Design review of the part built by this model. Coordinates are the model's own, in mm. A direction names the side the tool comes from. Round coordinates to 2 decimals unless told otherwise and drop trailing zeros. Write each loop counter-clockwise with the first axis right and the second up, starting at its lowest first coordinate (ties: lowest second). Pieces come first, ordered by that corner, then holes. Notation, with made-up numbers: M 21,16.25 L 70,16.25 A11 cw 70,21.25 Z; hole C 7.25,27.5 d5. An arc over 180 degrees is marked long. One line per question, with ' | ' between items. Start each with the question number.
Item 1: Machinability: for faces 1 (the face through (-11.986, 1.972, -1.586)), 2 (the face through (-2.645, 1.972, -13.127)), 3 (the face through (-11.15, 1.97, -7.41)), 4 (the face through (11.995, 1.972, -5.952)), which of the approach directions +Z, -Z, +X, -X, +Y, -Y give a long, thin tool a straight path to every point of the face, cutting with its end or side? Answer none if there is none.
Item 2: Insertion check: pin 1 Ø1 at (x, y) = (13.5, 1) entering from -Z; pin 2 Ø1.2 at (x, y) = (22.5, 1.5) entering from +Z; pin 3 Ø3.5 at (x, z) = (4.5, 0) entering from -Y; pin 4 Ø1 at (x, y) = (16, 1.5) entering from -Z. Each pin has a flat end and moves straight along its axis. Give the tip position at first contact, or say it passes through.
Item 3: Add section A-A, the plane y = 3.2. Give the number of separate pieces and of enclosed holes in the cut face, and give its area (3 significant figures).
Item 4: Add section B-B, the plane x = 19. State the section outline as (y, z) points.
Item 5: Draft analysis for pull direction X (two halves, no side actions). For faces 5 (the face through (10.046, 1.972, -8.853)), 6 (the face through (2.664, 1.972, -13.159)), 7 (the face through (-13.159, 1.972, -2.664)), state which applies: released by +X, released by -X, zero draft, split by the parting line, or undercut.
Item 6: For L1, parallel to X at y = 2.1, z = 0; L2, parallel to Z at x = 21, y = 3.3; L3, parallel to Z at x = -11.5, y = 1.75, list the stretches that pass through material, from the lowest coordinate up.
Item 7: Add section C-C, the plane z = -3. State the section outline as (x, y) points, and give its area (3 significant figures).
```python
from build123d import *

# Parameters (mm, degrees)
SKETCH_2_R          = 1.75
EXTRUDE_1_DEPTH     = 4
SKETCH_3_R          = 2.4
SKETCH_3_R_2        = 1.3
CUT_EXTRUDE_1_DEPTH = 38.993706757


with BuildPart() as part:
    # 草图2 → 凸台-拉伸1 (new body)
    with BuildSketch(Plane(origin=(0, 0, 0), x_dir=(1, 0, 0), z_dir=(0, 1, 0))):
        with BuildLine():
            ThreePointArc((30.75, -4.085109489), (34.835109489, 0), (30.75, 4.085109489))
            Line((30.75, 4.085109489), (14.048088143, 4.085109489))
            ThreePointArc((14.048088143, 4.085109489), (12.709169027, 4.272836063), (11.365584201, 4.122086336))
            ThreePointArc((11.365584201, 4.122086336), (11.169703548, 4.626642697), (10.951436862, 5.12192646))
            ThreePointArc((10.951436862, 5.12192646), (12.008090957, 5.965388247), (12.82210701, 7.044889767))
            ThreePointArc((12.82210701, 7.044889767), (12.669951657, 7.315), (12.51210701, 7.581825517))
            ThreePointArc((12.51210701, 7.581825517), (11.170223244, 7.416617696), (9.911436862, 6.9232593))
            ThreePointArc((9.911436862, 6.9232593), (9.591641884, 7.359925677), (9.252623584, 7.781841479))
            ThreePointArc((9.252623584, 7.781841479), (10.05496909, 8.870045207), (10.561852666, 10.123446462))
            ThreePointArc((10.561852666, 10.123446462), (10.344972209, 10.344972209), (10.123446462, 10.561852666))
            ThreePointArc((10.123446462, 10.561852666), (8.870045207, 10.05496909), (7.781841479, 9.252623584))
            ThreePointArc((7.781841479, 9.252623584), (7.359925677, 9.591641884), (6.9232593, 9.911436862))
            ThreePointArc((6.9232593, 9.911436862), (7.416617696, 11.170223244), (7.581825517, 12.51210701))
            ThreePointArc((7.581825517, 12.51210701), (7.315, 12.669951657), (7.044889767, 12.82210701))
            ThreePointArc((7.044889767, 12.82210701), (5.965388247, 12.008090957), (5.12192646, 10.951436862))
            ThreePointArc((5.12192646, 10.951436862), (4.626642697, 11.169703548), (4.122086336, 11.365584201))
            ThreePointArc((4.122086336, 11.365584201), (4.272836063, 12.709169027), (4.085109489, 14.048088143))
            ThreePointArc((4.085109489, 14.048088143), (3.78652263, 14.131494839), (3.486235477, 14.208555951))
            ThreePointArc((3.486235477, 14.208555951), (2.654199937, 13.14288127), (2.112960617, 11.903927815))
            ThreePointArc((2.112960617, 11.903927815), (1.578061664, 11.986568374), (1.04, 12.04518576))
            ThreePointArc((1.04, 12.04518576), (0.837867713, 13.382005944), (0.31, 14.626715284))
            ThreePointArc((0.31, 14.626715284), (0, 14.63), (-0.31, 14.626715284))
            ThreePointArc((-0.31, 14.626715284), (-0.837867713, 13.382005944), (-1.04, 12.04518576))
            ThreePointArc((-1.04, 12.04518576), (-1.578061664, 11.986568374), (-2.112960617, 11.903927815))
            ThreePointArc((-2.112960617, 11.903927815), (-2.654199937, 13.14288127), (-3.486235477, 14.208555951))
            ThreePointArc((-3.486235477, 14.208555951), (-3.78652263, 14.131494839), (-4.085109489, 14.048088143))
            ThreePointArc((-4.085109489, 14.048088143), (-4.272836063, 12.709169027), (-4.122086336, 11.365584201))
            ThreePointArc((-4.122086336, 11.365584201), (-4.626642697, 11.169703548), (-5.12192646, 10.951436862))
            ThreePointArc((-5.12192646, 10.951436862), (-5.965388247, 12.008090957), (-7.044889767, 12.82210701))
            ThreePointArc((-7.044889767, 12.82210701), (-7.315, 12.669951657), (-7.581825517, 12.51210701))
            ThreePointArc((-7.581825517, 12.51210701), (-7.416617696, 11.170223244), (-6.9232593, 9.911436862))
            ThreePointArc((-6.9232593, 9.911436862), (-7.359925677, 9.591641884), (-7.781841479, 9.252623584))
            ThreePointArc((-7.781841479, 9.252623584), (-8.870045207, 10.05496909), (-10.123446462, 10.561852666))
            ThreePointArc((-10.123446462, 10.561852666), (-10.344972209, 10.344972209), (-10.561852666, 10.123446462))
            ThreePointArc((-10.561852666, 10.123446462), (-10.05496909, 8.870045207), (-9.252623584, 7.781841479))
            ThreePointArc((-9.252623584, 7.781841479), (-9.591641884, 7.359925677), (-9.911436862, 6.9232593))
            ThreePointArc((-9.911436862, 6.9232593), (-11.170223244, 7.416617696), (-12.51210701, 7.581825517))
            ThreePointArc((-12.51210701, 7.581825517), (-12.669951657, 7.315), (-12.82210701, 7.044889767))
            ThreePointArc((-12.82210701, 7.044889767), (-12.008090957, 5.965388247), (-10.951436862, 5.12192646))
            ThreePointArc((-10.951436862, 5.12192646), (-11.169703548, 4.626642697), (-11.365584201, 4.122086336))
            ThreePointArc((-11.365584201, 4.122086336), (-12.709169027, 4.272836063), (-14.048088143, 4.085109489))
            ThreePointArc((-14.048088143, 4.085109489), (-14.131494839, 3.78652263), (-14.208555951, 3.486235477))
            ThreePointArc((-14.208555951, 3.486235477), (-13.14288127, 2.654199937), (-11.903927815, 2.112960617))
            ThreePointArc((-11.903927815, 2.112960617), (-11.986568374, 1.578061664), (-12.04518576, 1.04))
            ThreePointArc((-12.04518576, 1.04), (-13.382005944, 0.837867713), (-14.626715284, 0.31))
            ThreePointArc((-14.626715284, 0.31), (-14.63, 0), (-14.626715284, -0.31))
            ThreePointArc((-14.626715284, -0.31), (-13.382005944, -0.837867713), (-12.04518576, -1.04))
            ThreePointArc((-12.04518576, -1.04), (-11.986568374, -1.578061664), (-11.903927815, -2.112960617))
            ThreePointArc((-11.903927815, -2.112960617), (-13.14288127, -2.654199937), (-14.208555951, -3.486235477))
            ThreePointArc((-14.208555951, -3.486235477), (-14.131494839, -3.78652263), (-14.048088143, -4.085109489))
            ThreePointArc((-14.048088143, -4.085109489), (-12.709169027, -4.272836063), (-11.365584201, -4.122086336))
            ThreePointArc((-11.365584201, -4.122086336), (0.019655269, -12.089984023), (11.378927035, -4.085109489))
            Line((11.378927035, -4.085109489), (30.75, -4.085109489))
        make_face()
        with Locations(Location((0, 0, 0), (0, 0, 270))):
            Circle(SKETCH_2_R, mode=Mode.SUBTRACT)
        with Locations(Location((30.75, 0, 0), (0, 0, 270))):
            Circle(SKETCH_2_R, mode=Mode.SUBTRACT)
    extrude(amount=EXTRUDE_1_DEPTH)

    # 草图3 → 切除-拉伸1 (cut, through all)
    with BuildSketch(Plane(origin=(0, 4, 0), x_dir=(1, 0, 0), z_dir=(0, 1, 0))):
        with Locations(Location((0, 0, 0), (0, 0, 270))):
            Circle(SKETCH_3_R)
        with Locations(Location((4.5, 0, 0), (0, 0, 270))):
            Circle(SKETCH_3_R_2)
        with Locations(Location((-4.5, 0, 0), (0, 0, 270))):
            Circle(SKETCH_3_R_2)
    extrude(amount=-CUT_EXTRUDE_1_DEPTH, mode=Mode.SUBTRACT)


solid = part.part
```
Computed values:
1) face 1: -X, +Y, -Y | face 2: -Z, +Y, -Y | face 3: +Y, -Y | face 4: +X, +Y, -Y
2) pin 1: stops at z = -4.26 | pin 2: stops at z = 4.09 | pin 3: stops at y = 0 | pin 4: stops at z = -4.09
3) separate pieces: 1 | enclosed holes: 4 | area: 650 mm^2
4) outline: M 0,-4.09 L 4,-4.09 L 4,4.09 L 0,4.09 Z
5) face 5: released by +X | face 6: undercut | face 7: released by -X
6) L1: x = -14.63 to -5.8, -3.2 to -2.4, 2.4 to 3.2, 5.8 to 29, 32.5 to 34.84 | L2: z = -4.09 to 4.09 | L3: z = -7.49 to -5.51, -4.15 to 4.15
7) outline: M -13.65,0 L 33.52,0 L 33.52,4 L -13.65,4 Z | area: 189 mm^2
